Source: CAD feature listing. Evaluate the final solid. Frame: model axes, mm. Face numbers are marked on the shaded views. Round coordinates to 2 decimals unless told otherwise and drop trailing zeros. Loops run counter-clockwise (first coordinate to the right, second up) from the corner with the lowest first, then second, coordinate; pieces in that order, holes last.
(1) Section B-B, the plane y = 7.5. Return the cut outline in (x, z).
(2) Section A-A, the plane x = 225. Return the cut outline in (y, z).
(3) Section C-C, the plane x = 105. Return the cut outline in (y, z).
(4) Material intervals for probe 1 along Z at (x, y) = (84, 4.5); probe 2 along Y at (x, z) = (225, -0.9); probe 3 along Z at (x, y) = (105, 12.1), sorted ascending.
(5) Mould query, pull axis Z, two halves, no side actions, for the marked faces 1, 2 and 3. Classes: pulls with the +Z half, pulls with the -Z half, needs draft (parallel to the pull), parting line crosses it, or undercut.
(6) First-contact query: pin 1 Ø1.5 at (x, y) = (101, -4.5) entering from -Z; pin 2 Ø1.5 at (x, z) = (199.5, 3.5) entering from -Y; pin 3 Ø6 at (x, y) = (16, 2.5) entering from +Z; pin 4 Ø12 at (x, y) = (155.5, 6.5) entering from -Z. Flat tips, straight axial feed; report the tip coordinate or a pass-through.
(7) Section D-D, the plane x = 150. Return the cut outline in (y, z).
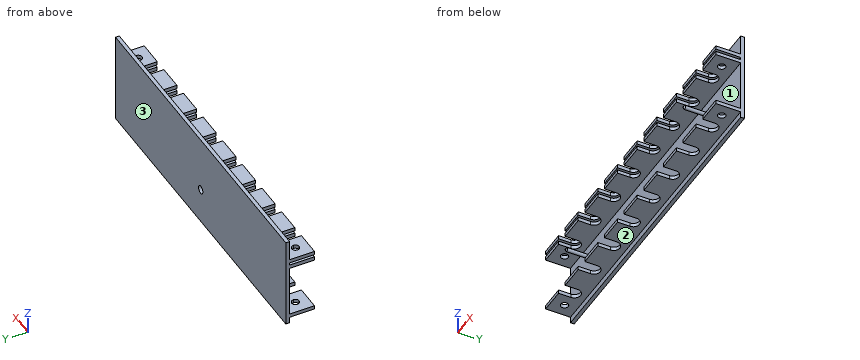
```python
from build123d import *

# Parameters (mm, degrees)
F0_W      = 30
F0_H      = 20
F1_DEPTH  = 3
F2_W      = 30
F2_H      = 21.6892715544
F2_H_2    = 3
F2_H_3    = 50
F3_DEPTH  = 3
F4_W      = 30
F4_H      = 3
F5_DEPTH  = 20
F10_W     = 240
F10_H     = 23
F11_DEPTH = 3
F12_W     = 10.1
F12_H     = 10
F13_DEPTH = 72
F15_D     = 6.6
F15_DEPTH = 21.5
F15_TIP   = 1.9828400428
F16_R     = 1.5
F17_DEPTH = 25
F18_SIZE  = 1
F20_DEPTH = 10
F22_DEPTH = 10
F23_R     = 3
F24_DEPTH = 60


# Not quite as in the source:
# - a feature names something its author has since deleted; it is built from what else it names


with BuildPart() as f1:
    # F0 (on Top) → F1 (new body)
    with BuildSketch(Plane.XY):
        Rectangle(F0_W, F0_H)
    extrude(amount=-F1_DEPTH)

    # F2 (on face) → F3 (join)
    with BuildSketch(Plane(origin=(0, 10, 0), x_dir=(-1, 0, 0), z_dir=(0, 1, 0))):
        with Locations((0, 10.8446357772)):
            Rectangle(F2_W, F2_H)
        with Locations((0, -1.5)):
            Rectangle(F2_W, F2_H_2)
        with Locations((0, -28)):
            Rectangle(F2_W, F2_H_3)
    extrude(amount=F3_DEPTH)

    # F4 (on face) → F5 (join)
    with BuildSketch(Plane.XZ.offset(-10)):
        with Locations((0, 3.5)):
            Rectangle(F4_W, F4_H)
    extrude(amount=F5_DEPTH)

    # F6: F1 across face


with BuildPart() as f1_1:
    add(f1.part)
    add(f1.part.mirror(Plane(origin=(15, 7.489162772, -9.8464985819), x_dir=(0, 1, 0), z_dir=(1, 0, 0))))

    # F7: F1 across face


with BuildPart() as f1_2:
    add(f1_1.part)
    add(f1_1.part.mirror(Plane(origin=(45, 7.489162772, -9.8464985819), x_dir=(0, 1, 0), z_dir=(1, 0, 0))))

    # F8: F1 across face


with BuildPart() as f1_3:
    add(f1_2.part)
    add(f1_2.part.mirror(Plane(origin=(105, 7.489162772, -9.8464985819), x_dir=(0, 1, 0), z_dir=(1, 0, 0))))

    # F10 (on offset) → F11 (join)
    with BuildSketch(Plane(origin=(0, 0, -48), x_dir=(1, 0, 0), z_dir=(0, 0, -1))):
        with Locations((105, -1.5)):
            Rectangle(F10_W, F10_H)
    extrude(amount=-F11_DEPTH)

    # F12 (on face) → F13 (cut)
    with BuildSketch(Plane(origin=(0, 0, -48), x_dir=(1, 0, 0), z_dir=(0, 0, -1))):
        with Locations((0, 5)):
            Rectangle(F12_W, F12_H)
        with BuildLine():
            Line((5.05, 0), (-5.05, 0))
            ThreePointArc((-5.05, 0), (0, -5.05), (5.05, 0))
        make_face()
        with BuildLine():
            Line((35.05, 10), (24.95, 10))
            Line((24.95, 10), (24.95, 0))
            ThreePointArc((24.95, 0), (30, -5.05), (35.05, 0))
            Line((35.05, 0), (35.05, 10))
        make_face()
        with BuildLine():
            Line((65.05, 10), (54.95, 10))
            Line((54.95, 10), (54.95, 0))
            ThreePointArc((54.95, 0), (60, -5.05), (65.05, 0))
            Line((65.05, 0), (65.05, 10))
        make_face()
        with BuildLine():
            Line((95.05, 10), (84.95, 10))
            Line((84.95, 10), (84.95, 0))
            ThreePointArc((84.95, 0), (90, -5.05), (95.05, 0))
            Line((95.05, 0), (95.05, 10))
        make_face()
        with BuildLine():
            Line((125.05, 10), (114.95, 10))
            Line((114.95, 10), (114.95, 0))
            ThreePointArc((114.95, 0), (120, -5.05), (125.05, 0))
            Line((125.05, 0), (125.05, 10))
        make_face()
        with BuildLine():
            Line((155.05, 0), (155.05, 10))
            Line((155.05, 10), (144.95, 10))
            Line((144.95, 10), (144.95, 0))
            ThreePointArc((144.95, 0), (150, -5.05), (155.05, 0))
        make_face()
        with BuildLine():
            Line((185.05, 0), (185.05, 10))
            Line((185.05, 10), (174.95, 10))
            Line((174.95, 10), (174.95, 0))
            ThreePointArc((174.95, 0), (180, -5.05), (185.05, 0))
        make_face()
        with BuildLine():
            Line((215.05, 0), (215.05, 10))
            Line((215.05, 10), (204.95, 10))
            Line((204.95, 10), (204.95, 0))
            ThreePointArc((204.95, 0), (210, -5.05), (215.05, 0))
        make_face()
    extrude(amount=-F13_DEPTH, mode=Mode.SUBTRACT)

    # F15
    with Locations(Plane.XZ.offset(-10)):
        with Locations((105, -24)):
            Hole(F15_D / 2, depth=F15_DEPTH)
            with Locations((0, 0, -(F15_DEPTH + F15_TIP / 2))):  # 118° drill point
                Cone(0, F15_D / 2, F15_TIP, mode=Mode.SUBTRACT)

    # F16 (on face) → F17 (join)
    with BuildSketch(Plane.XZ.offset(-10)):
        with Locations((15, -24)):
            Circle(F16_R)
        with Locations((195, -24)):
            Circle(F16_R)
    extrude(amount=F17_DEPTH)

    # F18
    f18_edges = [f1_3.edges().sort_by_distance(p)[0] for p in [
        (13.5, -15, -24),
        (193.5, -15, -24),
    ]]
    chamfer(f18_edges, length=F18_SIZE)

    # F19 (on face) → F20 (join)
    with BuildSketch(Plane.YZ.offset(225)):
        Polygon((13, 21.6892715544), (10, 21.6892715544), (10, 5), (-10, 5), (-10, 2), (10, 2), (10, 0), (-10, 0), (-10, -3), (10, -3), (10, -45), (-10, -45), (-10, -48), (10, -48), (10, -53), (13, -53), align=None)
    extrude(amount=F20_DEPTH)

    # F21 (on face) → F22 (join)
    with BuildSketch(Plane(origin=(-15, 0, 0), x_dir=(0, -1, 0), z_dir=(-1, 0, 0))):
        Polygon((-10, 5), (-10, 21.6892715544), (-13, 21.6892715544), (-13, -53), (-10, -53), (-10, -48), (10, -48), (10, -45), (-10, -45), (-10, -3), (10, -3), (10, 0), (-10, 0), (-10, 2), (10, 2), (10, 5), align=None)
    extrude(amount=F22_DEPTH)

    # F23 (on face) → F24 (cut)
    with BuildSketch(Plane.XY.offset(5)):
        with BuildLine():
            ThreePointArc((-15, -3), (-12.8786796564, -2.1213203436), (-12, 0))
            ThreePointArc((-12, 0), (-12.8786796564, 2.1213203436), (-15, 3))
            Line((-15, 3), (-15, -3))
        make_face()
        with BuildLine():
            Line((-15, -3), (-15, 3))
            ThreePointArc((-15, 3), (-18, 0), (-15, -3))
        make_face()
        with Locations((225, 0)):
            Circle(F23_R)
    extrude(amount=-F24_DEPTH, mode=Mode.SUBTRACT)


solid = f1_3.part
```
Output values:
1. outline: (-25, -48) - (235, -48) - (235, -45) - (-25, -45) - close; (-25, -3) - (235, -3) - (235, 0) - (-25, 0) - close; (-25, 2) - (235, 2) - (235, 5) - (-25, 5) - close; circle Ø3 at (15, -24); circle Ø3 at (195, -24)
2. outline: (-10, -48) - (-3, -48) - (-3, -45) - (-10, -45) - close; (-10, -3) - (-3, -3) - (-3, 0) - (-10, 0) - close; (-10, 2) - (-3, 2) - (-3, 5) - (-10, 5) - close; (3, -48) - (10, -48) - (10, -53) - (13, -53) - (13, 21.69) - (10, 21.69) - (10, 5) - (3, 5) - (3, 2) - (10, 2) - (10, 0) - (3, 0) - (3, -3) - (10, -3) - (10, -45) - (3, -45) - close
3. outline: (-10, -48) - (10, -48) - (10, -53) - (13, -53) - (13, -27.3) - (10, -27.3) - (10, -45) - (-10, -45) - close; (-10, -3) - (10, -3) - (10, -20.7) - (13, -20.7) - (13, 21.69) - (10, 21.69) - (10, 5) - (-10, 5) - (-10, 2) - (10, 2) - (10, 0) - (-10, 0) - close
4. probe 1: z = -48 to -45, -3 to 0, 2 to 5
4. probe 2: y = -10 to -3, 3 to 13
4. probe 3: z = -53 to -27.3, -20.7 to 21.69
5. face 1: undercut
5. face 2: pulls with the -Z half
5. face 3: needs draft
6. pin 1: stops at z = -48
6. pin 2: stops at y = -10
6. pin 3: stops at z = 5
6. pin 4: stops at z = -53
7. outline: (5.05, -48) - (10, -48) - (10, -53) - (13, -53) - (13, 21.69) - (10, 21.69) - (10, 5) - (5.05, 5) - (5.05, 2) - (10, 2) - (10, 0) - (5.05, 0) - (5.05, -3) - (10, -3) - (10, -45) - (5.05, -45) - close
